Source: three-view drawing plus pictorial views. Frame: mm from the lowest corner of the part. A direction names the side the tool comes from. Give positions to 0.01 mm unless a question says otherwise; leave off trailing zeros. Write each loop counter-clockwise with the first axis right and the second up, starting at its lowest first coordinate (ties: lowest second). Pieces come first, ordered by that corner, then holes. Notation, with made-up numbers: M 0,50 L 10,50 A19 ccw 10,72 Z; hole C 58,88.5 d10. An arc over 180 degrees is marked long. Return JSON: item names as keys, results as strings.
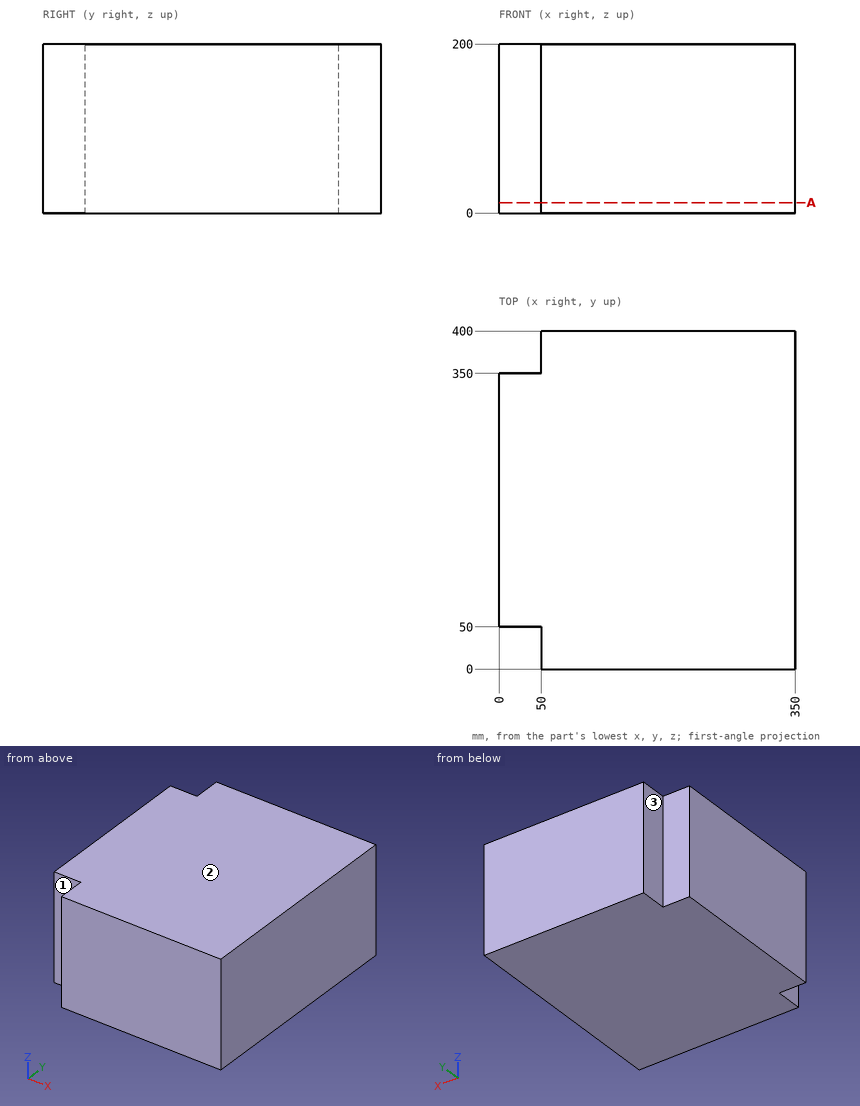
1) Contact query for flat-ended pins moving along their axis: pin 1 Ø15 at (x, z) = (16.5, 124.5) entering from +Y; pin 2 Ø15 at (y, z) = (25, 129.5) entering from -X; pin 3 Ø15 at (x, z) = (26.5, 73.5) entering from -Y. Output: stop coordinate, or through.
Numbers:
{"pin 1": "stops at y = 350", "pin 2": "stops at x = 50", "pin 3": "stops at y = 50"}
2) Set-up query: the marked faces 1, 2 and 3. Return all of +Z, -Z, +X, -X, +Y, -Y with unobstructed straight access to the full face (end or side cutting, diameter ignored); none if empty.
Numbers:
{"face 1": "+Z, -Z, -X, -Y", "face 2": "+Z, +X, -X, +Y, -Y", "face 3": "+Z, -Z, -X, +Y"}
3) Cut plane A-A, the plane z = 12.5. Return the cut outline in (x, y).
Numbers:
{"outline": "M 0,50 L 50,50 L 50,0 L 350,0 L 350,400 L 50,400 L 50,350 L 0,350 Z"}
4) Line query: line 1 (X direction, y = 39.5, z = 81). Output: solid intervals per line, ascending. Write a range as [from, to].
Numbers:
{"line 1": "x = [50, 350]"}
